Part print with two shaded views. Sizes in mm from the minimum x, y, z corner. Give positions to 0.01 mm unless a question says otherwise; leave off trailing zeros. Write each loop counter-clockwise with the first axis right and the second up, starting at its lowest first coordinate (ties: lowest second). Pieces come first, ordered by that corner, then holes. Notation, with made-up numbers: (61, 16) - (112, 16) arc R15 ccw to (112, 24) - close; hole circle Ø3 at (52.5, 53). An arc over 180 degrees is marked (long way). Answer as a JSON object with one key per item and string values. Group by question number.
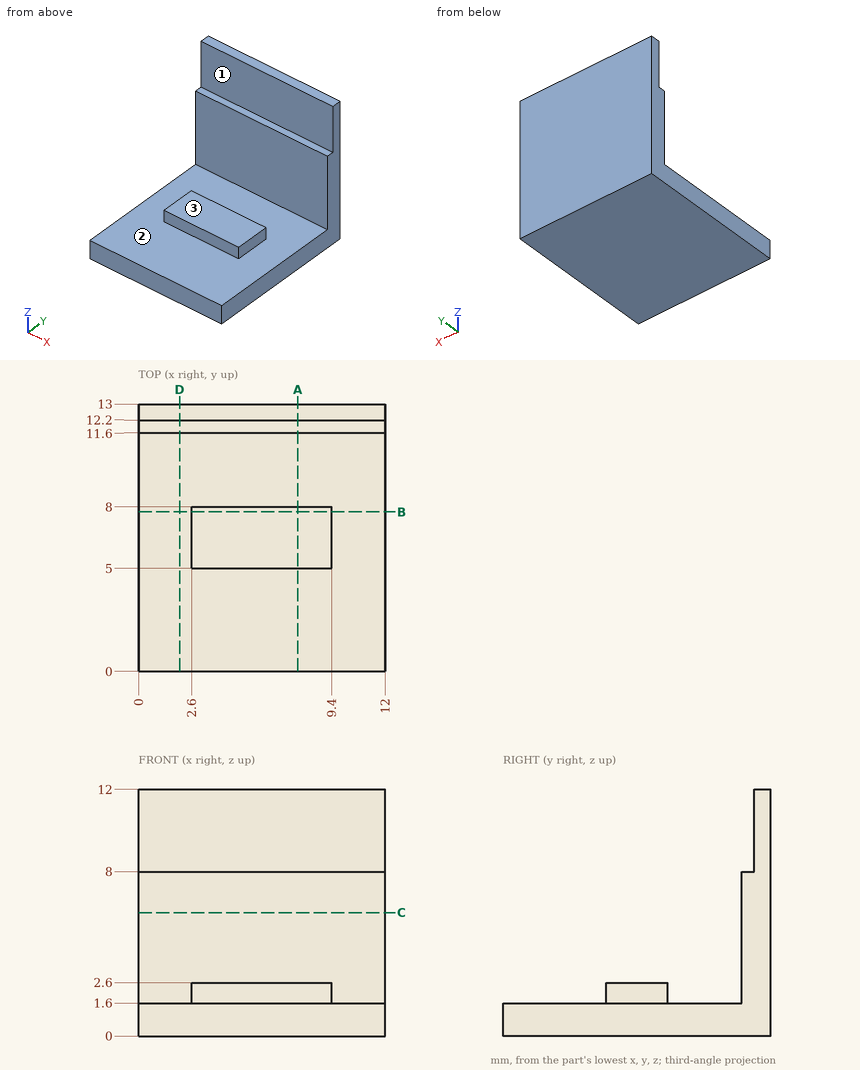
1) Saw through at C-C (z = 6). List the corners of the cut face in (x, y).
2) Two-plate mould, pull along Y, no slides. Class the marked faces 1, 2 and 3: +Y half, -Y half, draft (parallel to the pull), parting line (faces both ways), or undercut.
3) Saw through at B-B (y = 7.75). List the corners of the cut face in (x, z).
4) Drill centre lines: line 1 along Y through (x, z) = (9, 2); line 2 along Z through (x, y) = (5, 7); line 3 along Y through (x, z) = (10.5, 5.5). Where is each one in solid material? Low to high. Write a range as from..to.
5) Drop flat-ended pins along their axis: P1, Ø0.5, axis at y = 6, z = 2, coming from the +X side; P2, Ø1.2, axis at x = 4, z = 10, coming from the -Y side; P3, Ø2.5, axis at x = 7, y = 6, coming from the +Z side. Give the stop position or say it passes through.
6) Saw through at A-A (x = 7.75). List the corners of the cut face in (y, z), and give its area (3 significant figures).
7) Saw through at D-D (x = 2). List the corners of the cut face in (y, z), and give its area (3 significant figures).
Checks:
{
 "1": {"outline": "(0, 11.6) - (12, 11.6) - (12, 13) - (0, 13) - close"},
 "2": {"face 1": "-Y half", "face 2": "undercut", "face 3": "draft"},
 "3": {"outline": "(0, 0) - (12, 0) - (12, 1.6) - (9.4, 1.6) - (9.4, 2.6) - (2.6, 2.6) - (2.6, 1.6) - (0, 1.6) - close"},
 "4": {"line 1": "5..8, 11.6..13", "line 2": "0..2.6", "line 3": "11.6..13"},
 "5": {"P1": "x = 9.4", "P2": "y = 12.2", "P3": "z = 2.6"},
 "6": {"outline": "(0, 0) - (13, 0) - (13, 12) - (12.2, 12) - (12.2, 8) - (11.6, 8) - (11.6, 1.6) - (8, 1.6) - (8, 2.6) - (5, 2.6) - (5, 1.6) - (0, 1.6) - close", "area": "36.0 mm2"},
 "7": {"outline": "(0, 0) - (13, 0) - (13, 12) - (12.2, 12) - (12.2, 8) - (11.6, 8) - (11.6, 1.6) - (0, 1.6) - close", "area": "33.0 mm2"}
}
